For this review, take the finished solid that the model builds, in its own axes (mm). Coordinates: 2 decimals unless noted, no trailing zeros. Loops run counter-clockwise (first coordinate to the right, second up) from the corner with the lowest first, then second, coordinate; pieces in that order, holes last. Notation, with made-up numbers: (-22, -16) - (35, -16) arc R27 cw to (35, 11) - close; hole circle Ø10 at (-33, 10). An arc over 180 degrees is marked (long way). Use one line per item in the form item = value. Start each with the question number.
1. To check wall thickness, follow probe 1 along Z at (x, y) = (0, -7.75) (1 decimal); probe 2 along X at (y, z) = (-8, 0.5). State the ranges of each line that lie inside material, in increasing order.
2. Add section B-B on y = -3.75. Give the boundary of the cut face in (x, z) (3 decimals), and give its area (3 significant figures).
3. Draft analysis for pull direction X (two halves, no side actions). For faces 1 (the face through (-0.045, -4.719, -0.205)), 2 (the face through (0, 0, 0)), 3 (the face through (-0.69, -4.78, -3.1)), state which applies: +X half, -X half, draft (parallel to the pull), parting line (faces both ways), or undercut.
4. For pin 1 Ø1.5 at (x, y) = (-1, -7.5) entering from -Z, flat-tipped, find the tip position at first contact; note if it passes through.
```python
from build123d import *

# Parameters (mm, degrees)
F0_R     = 3.175
F1_DEPTH = 12.7
F2_SIZE  = 3
F4_D     = 2.413
F4_DEPTH = 6.35
F4_START = 1.0315
F4_TIP   = 0.7249383369


with BuildPart() as f1:
    # F0 (on Front) → F1 (new body)
    with BuildSketch(Plane.XZ):
        Circle(F0_R)
    extrude(amount=F1_DEPTH)

    # F2
    f2_edges = [f1.edges().sort_by_distance(p)[0] for p in [
        (-3.175, -12.7, 0),
    ]]
    chamfer(f2_edges, length=F2_SIZE)

    # F4
    # its depths count from where the whole tool has entered the part; down to there all is cleared
    with Locations(Plane.XZ.offset(12.7).offset(-F4_START)):
        with Locations((0, 0)):
            Hole(F4_D / 2, depth=F4_DEPTH)
            with Locations((0, 0, -(F4_DEPTH + F4_TIP / 2))):  # 118° drill point
                Cone(0, F4_D / 2, F4_TIP, mode=Mode.SUBTRACT)


solid = f1.part
```
Conclusion:
q1.probe_1 = -3.2 to -1.2, 1.2 to 3.2
q1.probe_2 = -3.14 to -1.1, 1.1 to 3.14
q2.outline = circle Ø6.35 at (0, 0)
q2.area = 31.7 mm^2
q3.face_1 = undercut
q3.face_2 = draft
q3.face_3 = parting line
q4.pin_1 = -3.17
